Part print with two shaded views. Sizes in mm from the minimum x, y, z corner. A direction names the side the tool comes from. Give positions to 0.01 mm unless a question says otherwise; leave off trailing zeros. Loops run counter-clockwise (first coordinate to the right, second up) from the corner with the lowest first, then second, coordinate; pieces in that order, holes last. Notation, with made-up numbers: M 86.25,-4 L 105.25,-4 A9 cw 105.25,13 Z; hole C 1,82.25 d2. An arc over 180 degrees is marked long. Answer in a Markdown table with one row per item.
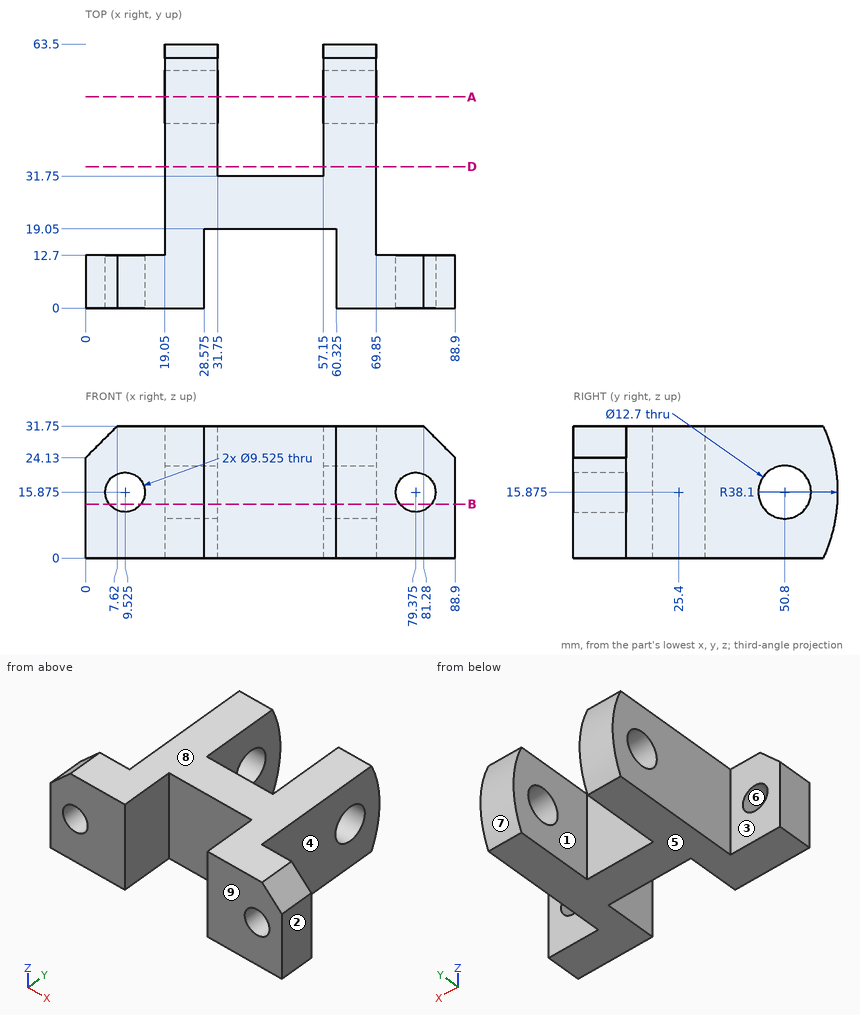
Q1. 3-axis set-ups, long thin cutter, end or side, ignore diameter. For the marked faces 1, 2, 3, 4 and 5: which of +Z, -Z, +X, -X, +Y, -Y reach the whole face in a straight line?
Reported:
| item | result |
|---|---|
| face 1 | +Z, -Z, +Y |
| face 2 | +Z, -Z, +X, +Y, -Y |
| face 3 | +Z, -Z, -X, +Y |
| face 4 | +Z, -Z, +X, +Y |
| face 5 | -Z, +X, -X, +Y, -Y |
Q2. Probe probe 1 along X at (y, z) = (32, 23); probe 2 along X at (y, z) = (17, 10.5) (3 decimals); probe 3 along Y at (x, z) = (14, 25). List the from-to ranges inside material, lowest first.
Reported:
| item | result |
|---|---|
| probe 1 | 19.05 to 31.75, 57.15 to 69.85 |
| probe 2 | 19.05 to 28.575, 60.325 to 69.85 |
| probe 3 | 0 to 12.7 |
Q3. Saw through at B-B (z = 13). Give the number of separate pieces and of enclosed holes in the cut face, and give its area (3 significant figures).
Reported:
| item | result |
|---|---|
| separate pieces | 5 |
| enclosed holes | 0 |
| area | 1,820 mm² |
Q4. Saw through at A-A (y = 50.8). Give the cut face in (x, z) (3 decimals), and give its area (3 significant figures).
Reported:
| item | result |
|---|---|
| outline | M 19.05,0 L 31.75,0 L 31.75,9.525 L 19.05,9.525 Z; M 19.05,22.225 L 31.75,22.225 L 31.75,31.75 L 19.05,31.75 Z; M 57.15,0 L 69.85,0 L 69.85,9.525 L 57.15,9.525 Z; M 57.15,22.225 L 69.85,22.225 L 69.85,31.75 L 57.15,31.75 Z |
| area | 484 mm² |
Q5. Drop flat-ended pins along their axis: pin 1 (15 mm diameter, centred on x = 79.375, z = 15.875, fed in from +Y); pin 2 (16 mm diameter, centred on y = 47, z = 21.5, fed in from +X); pin 3 (1 mm diameter, centred on y = 27.5, z = 4, fed in from -X). Give the stop position or say it passes through.
Reported:
| item | result |
|---|---|
| pin 1 | y = 12.7 |
| pin 2 | x = 69.85 |
| pin 3 | x = 19.05 |
Q6. Saw through at D-D (y = 34). Give the cut face in (x, z).
Reported:
| item | result |
|---|---|
| outline | M 19.05,0 L 31.75,0 L 31.75,31.75 L 19.05,31.75 Z; M 57.15,0 L 69.85,0 L 69.85,31.75 L 57.15,31.75 Z |
Q7. Mould opens along Z. For the marked faces 6, 7, 8 and 9 say: released by +Z, released by -Z, zero draft, split by the parting line, or undercut.
Reported:
| item | result |
|---|---|
| face 6 | undercut |
| face 7 | split by the parting line |
| face 8 | released by +Z |
| face 9 | zero draft |
